Design review of the part shown in the three views and the two pictorial views. Dimensions are in mm from the part's minimum x, y and z. A direction names the side the tool comes from. Coordinates: 2 decimals unless noted, no trailing zeros. Order: outer loops, then holes, each group sorted by start corner. A loop starts at its lowest first (then second) coordinate and runs counter-clockwise, first axis right, second up. Notation, with made-up numbers: (-12.75, 3.5) - (19.25, 3.5) arc R9 ccw to (19.25, 8.5) - close; hole circle Ø10 at (50, -14). An arc over 180 degrees is marked (long way). One line per item, written item: value. Start each with the question number.
(1) Consider section A-A on z = 59. Write out the cut boundary in (x, y) (1 decimal).
(2) Clearance check with flat-ended pins moving along their axes: pin 1 (3 mm diameter, centred on y = 9.5, z = 59, fed in from +X); pin 2 (5 mm diameter, centred on x = 16, y = 1.5, fed in from +Z); pin 3 (2 mm diameter, centred on y = 5.5, z = 63, fed in from -X); pin 4 (6 mm diameter, centred on x = 76.02, z = 22.16, fed in from +Y). State where each tip first meets the part, or that it passes through.
(3) Mouldability with a two-part tool opening along X and no side actions: class the marked faces 3, 4 and 5 as released by +X, released by -X, zero draft, split by the parting line, or undercut.
(4) Consider section C-C on z = 26. Write out the cut boundary in (x, y).
(5) To check wall thickness, follow line 1 along X through (y, z) = (4.5, 85); line 2 along X through (y, z) = (4, 22) (1 decimal); line 3 along X through (y, z) = (5.25, 13.5) (1 decimal). State the ranges of each line that lie inside material, in increasing order.
(6) Consider section B-B on y = 10.5. Count the separate pieces of the cut face and the enclosed holes in it, then the cut area to 3 significant figures.
(7) For the marked faces 1 and 2, list the 3-axis set-ups (+Z, -Z, +X, -X, +Y, -Y) from which the entire face can be reached by the end or side of a thin tool; tool diameter is ignored.
(8) Consider section D-D on x = 62.5. Write out the cut boundary in (y, z) (1 decimal).
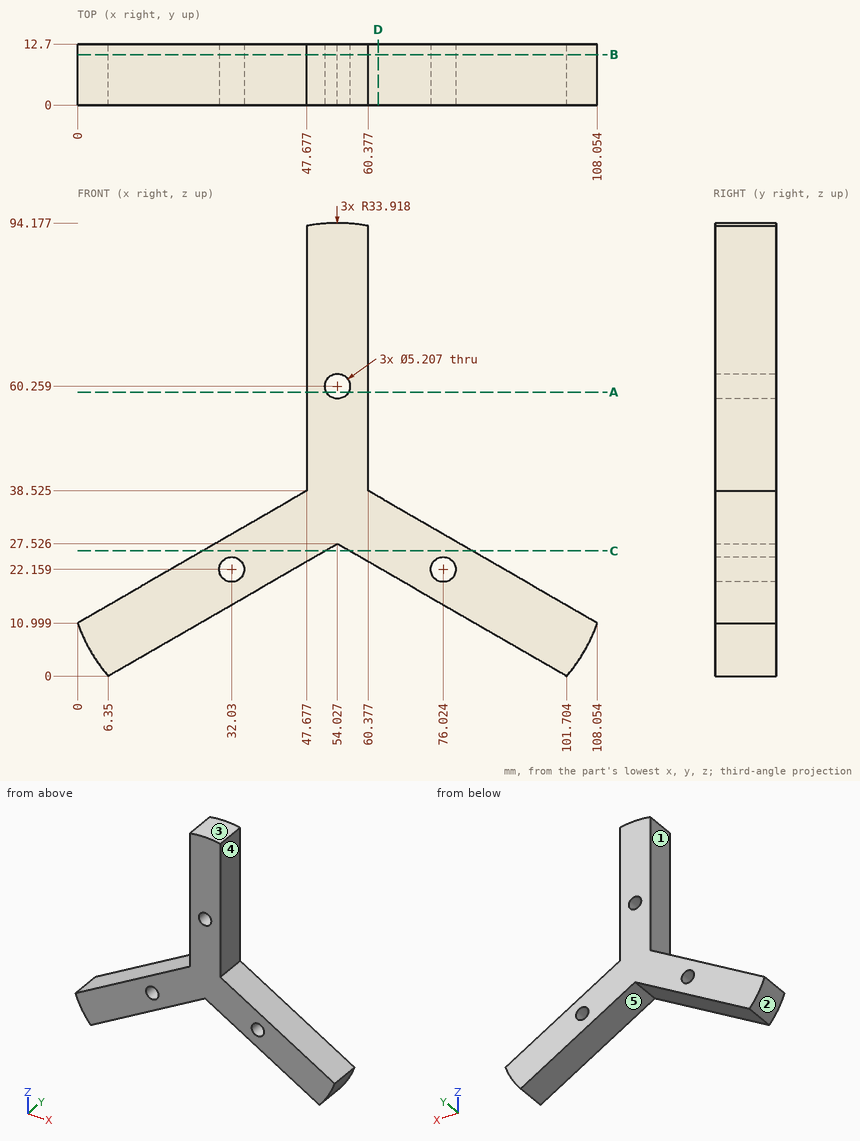
Geometry check:
1. outline: (47.7, 0) - (51.7, 0) - (51.7, 12.7) - (47.7, 12.7) - close; (56.3, 0) - (60.4, 0) - (60.4, 12.7) - (56.3, 12.7) - close
2. pin 1: stops at x = 60.38
2. pin 2: stops at z = 21.68
2. pin 3: stops at x = 47.68
2. pin 4: stops at y = 12.7
3. face 3: split by the parting line
3. face 4: released by +X
3. face 5: undercut
4. outline: (25.98, 0) - (51.38, 0) - (51.38, 12.7) - (25.98, 12.7) - close; (56.67, 0) - (82.07, 0) - (82.07, 12.7) - (56.67, 12.7) - close
5. line 1: x = 47.68 to 60.38
5. line 2: x = 19.1 to 29.4, 34.6 to 44.5, 63.6 to 73.4, 78.6 to 89
5. line 3: x = 4.3 to 29.7, 78.3 to 103.7
6. separate pieces: 1
6. enclosed holes: 3
6. area: 2,120 mm^2
7. face 1: +Z, -X, +Y, -Y
7. face 2: -Z, -X, +Y, -Y
8. outline: (0, 22.6) - (12.7, 22.6) - (12.7, 37.3) - (0, 37.3) - close
